from build123d import *

# Parameters (mm, degrees)
F1_DEPTH = 2


with BuildPart() as f1:
    # F0 (on Top) → F1 (new body)
    with BuildSketch(Plane.XY):
        with BuildLine():
            add(Edge.make_bspline(
                [(-8.3521283749, -0.7617495372), (-8.5671938563, -0.5078146578), (-8.7835969282, -0.2539073289), (-9, 0)],
                knots=[0.9592497634, 0.9592497634, 0.9592497634, 0.9592497634, 1, 1, 1, 1], degree=3))
            Line((-9, 0), (-8, 0))
            ThreePointArc((-8, 0), (-9.9077091013, 0.4196000327), (-8.3521283749, -0.7617495372))
        make_face()
        with BuildLine():
            Line((-8, 0), (-9, 0))
            add(Edge.make_bspline(
                [(-8.3521283749, -0.7617495372), (-8.5671938563, -0.5078146578), (-8.7835969282, -0.2539073289), (-9, 0)],
                knots=[0.9592497634, 0.9592497634, 0.9592497634, 0.9592497634, 1, 1, 1, 1], degree=3))
            ThreePointArc((-8.3521283749, -0.7617495372), (-8.0922908987, -0.4196000327), (-8, 0))
        make_face()
        with BuildLine():
            Line((-1.5, 0), (-8, 0))
            ThreePointArc((-8, 0), (-8.0922908987, -0.4196000327), (-8.3521283749, -0.7617495372))
            add(Edge.make_bspline(
                [(-3.5, -9.5), (-3.6213752497, -6.556436521), (-5.8997934607, -3.6573019366), (-8.3521283749, -0.7617495372)],
                knots=[0.4945855722, 0.4945855722, 0.4945855722, 0.4945855722, 0.9592497634, 0.9592497634, 0.9592497634, 0.9592497634], degree=3))
            Line((-3.5, -9.5), (0, -9.5))
            Line((0, -9.5), (0, -1.5))
            ThreePointArc((0, -1.5), (-1.0606601718, -1.0606601718), (-1.5, 0))
        make_face()
        with BuildLine():
            Line((0, 0), (-1.5, 0))
            ThreePointArc((-1.5, 0), (-1.0606601718, -1.0606601718), (0, -1.5))
            Line((0, -1.5), (0, 0))
        make_face()
        with BuildLine():
            ThreePointArc((1.5, 0), (0, 1.5), (-1.5, 0))
            Line((-1.5, 0), (0, 0))
            Line((0, 0), (1.5, 0))
        make_face()
        with BuildLine():
            Line((1.5, 0), (0, 0))
            Line((0, 0), (0, -1.5))
            ThreePointArc((0, -1.5), (1.0606601718, -1.0606601718), (1.5, 0))
        make_face()
        with BuildLine():
            Line((8, 0), (1.5, 0))
            ThreePointArc((1.5, 0), (1.0606601718, -1.0606601718), (0, -1.5))
            Line((0, -1.5), (0, -9.5))
            Line((0, -9.5), (3.5, -9.5))
            add(Edge.make_bspline(
                [(3.5, -9.5), (3.6213752497, -6.556436521), (5.8997934607, -3.6573019366), (8.3521283749, -0.7617495372)],
                knots=[0.4945855722, 0.4945855722, 0.4945855722, 0.4945855722, 0.9592497634, 0.9592497634, 0.9592497634, 0.9592497634], degree=3))
            ThreePointArc((8.3521283749, -0.7617495372), (8.0922908987, -0.4196000327), (8, 0))
        make_face()
        with BuildLine():
            Line((9, 0), (8, 0))
            ThreePointArc((8, 0), (8.0922908987, -0.4196000327), (8.3521283749, -0.7617495372))
            add(Edge.make_bspline(
                [(8.3521283749, -0.7617495372), (8.5671938563, -0.5078146578), (8.7835969282, -0.2539073289), (9, 0)],
                knots=[0.9592497634, 0.9592497634, 0.9592497634, 0.9592497634, 1, 1, 1, 1], degree=3))
        make_face()
        with BuildLine():
            ThreePointArc((10, 0), (9, 1), (8, 0))
            Line((8, 0), (9, 0))
            add(Edge.make_bspline(
                [(8.3521283749, -0.7617495372), (8.5671938563, -0.5078146578), (8.7835969282, -0.2539073289), (9, 0)],
                knots=[0.9592497634, 0.9592497634, 0.9592497634, 0.9592497634, 1, 1, 1, 1], degree=3))
            ThreePointArc((8.3521283749, -0.7617495372), (9.4196000327, -0.9077091013), (10, 0))
        make_face()
        with BuildLine():
            Line((0, -9.5), (-3.5, -9.5))
            add(Edge.make_bspline(
                [(-7.4128937144, -18.1904901425), (-5.3105671576, -15.277222995), (-3.3817599302, -12.3675298477), (-3.5, -9.5)],
                knots=[0.0419238759, 0.0419238759, 0.0419238759, 0.0419238759, 0.4945855722, 0.4945855722, 0.4945855722, 0.4945855722], degree=3))
            ThreePointArc((-7.4128937144, -18.1904901425), (-7.1091840017, -18.5456357659), (-7, -19))
            Line((-7, -19), (-1.5, -19))
            ThreePointArc((-1.5, -19), (-1.0606601718, -17.9393398282), (0, -17.5))
            Line((0, -17.5), (0, -9.5))
        make_face()
        with BuildLine():
            Line((3.5, -9.5), (0, -9.5))
            Line((0, -9.5), (0, -17.5))
            ThreePointArc((0, -17.5), (1.0606601718, -17.9393398282), (1.5, -19))
            Line((1.5, -19), (7, -19))
            ThreePointArc((7, -19), (7.1091840017, -18.5456357659), (7.4128937144, -18.1904901425))
            add(Edge.make_bspline(
                [(7.4128937144, -18.1904901425), (5.3105671576, -15.277222995), (3.3817599302, -12.3675298477), (3.5, -9.5)],
                knots=[0.0419238759, 0.0419238759, 0.0419238759, 0.0419238759, 0.4945855722, 0.4945855722, 0.4945855722, 0.4945855722], degree=3))
        make_face()
        with BuildLine():
            Line((0, -19), (0, -17.5))
            ThreePointArc((0, -17.5), (-1.0606601718, -17.9393398282), (-1.5, -19))
            Line((-1.5, -19), (0, -19))
        make_face()
        with BuildLine():
            ThreePointArc((1.5, -19), (1.0606601718, -17.9393398282), (0, -17.5))
            Line((0, -17.5), (0, -19))
            Line((0, -19), (1.5, -19))
        make_face()
        with BuildLine():
            Line((1.5, -19), (0, -19))
            Line((0, -19), (-1.5, -19))
            ThreePointArc((-1.5, -19), (0, -20.5), (1.5, -19))
        make_face()
        with BuildLine():
            add(Edge.make_bspline(
                [(-8, -19), (-7.8038017674, -18.7301531618), (-7.6076035348, -18.4603063237), (-7.4128937144, -18.1904901425)],
                knots=[0, 0, 0, 0, 0.0419238759, 0.0419238759, 0.0419238759, 0.0419238759], degree=3))
            ThreePointArc((-7.4128937144, -18.1904901425), (-8.8908159983, -19.4543642341), (-7, -19))
            Line((-7, -19), (-8, -19))
        make_face()
        with BuildLine():
            ThreePointArc((-7, -19), (-7.1091840017, -18.5456357659), (-7.4128937144, -18.1904901425))
            add(Edge.make_bspline(
                [(-8, -19), (-7.8038017674, -18.7301531618), (-7.6076035348, -18.4603063237), (-7.4128937144, -18.1904901425)],
                knots=[0, 0, 0, 0, 0.0419238759, 0.0419238759, 0.0419238759, 0.0419238759], degree=3))
            Line((-8, -19), (-7, -19))
        make_face()
        with BuildLine():
            add(Edge.make_bspline(
                [(8, -19), (7.8038017674, -18.7301531618), (7.6076035348, -18.4603063237), (7.4128937144, -18.1904901425)],
                knots=[0, 0, 0, 0, 0.0419238759, 0.0419238759, 0.0419238759, 0.0419238759], degree=3))
            ThreePointArc((7.4128937144, -18.1904901425), (7.1091840017, -18.5456357659), (7, -19))
            Line((7, -19), (8, -19))
        make_face()
        with BuildLine():
            ThreePointArc((9, -19), (8.4543642341, -18.1091840017), (7.4128937144, -18.1904901425))
            add(Edge.make_bspline(
                [(8, -19), (7.8038017674, -18.7301531618), (7.6076035348, -18.4603063237), (7.4128937144, -18.1904901425)],
                knots=[0, 0, 0, 0, 0.0419238759, 0.0419238759, 0.0419238759, 0.0419238759], degree=3))
            Line((8, -19), (7, -19))
            ThreePointArc((7, -19), (8, -20), (9, -19))
        make_face()
    extrude(amount=F1_DEPTH)


solid = f1.part
Could you check a few things on this model? Use its own coordinates, in mm. A direction names the side the tool comes from. Round coordinates to 2 decimals unless told otherwise and drop trailing zeros. Order: outer loops, then holes, each group sorted by start corner. A loop starts at its lowest first (then second) coordinate and runs counter-clockwise, first axis right, second up.
(1) Imagine slicing it at A-A (x = 1.75). Write out the boundary of the cut face in (y, z).
Response values:
outline: (-19, 0) - (0, 0) - (0, 2) - (-19, 2) - close
(2) Please list where these lines run through material, in increasing order: line 1 along Y through (x, z) = (-5.25, 0.55); line 2 along Y through (x, z) = (8.25, 1.8); line 3 along X through (y, z) = (-5.5, 0.9).
Response values:
line 1: y = -19 to -14.97, -4.8 to 0
line 2: y = -19.97 to -18.03, -0.88 to 0.66
line 3: x = -4.82 to 4.82
(3) I'm going to push a flat-ended pin straight in: pin 1 (0.6 mm diameter, centred on x = -4.5, z = 1, fed in from +Y). Where does the tip first touch, or does it pass through?
Response values:
pin 1: stops at y = 0
(4) Which directions (+Z, -Z, +X, -X, +Y, -Y) give clear straight access to the entire face, cutting with the end or side of a thin tool? Please do faces 4 (the flat face through (5, 0, 1)), 5 (the cylindrical face through (-10, 0, 1)), 6 (the flat face through (-4, -19, 1)).
Response values:
face 4: +Z, -Z, +Y
face 5: +Z, -Z
face 6: +Z, -Z, -Y
(5) If we mould it in two halves opening along Y, with no side actions, what happens to faces 1 (the cylindrical face through (-9, -19, 1)), 2 (the flat face through (0, -9, 2)), 3 (the flat face through (4, -19, 1))? For each: released by +Y, released by -Y, zero draft, split by the parting line, or undercut.
Response values:
face 1: undercut
face 2: zero draft
face 3: released by -Y
